```python
from build123d import *

# Parameters (mm, degrees)
SKETCH1_R           = 1.5
BOSS_EXTRUDE1_DEPTH = 2


with BuildPart() as part:
    # Sketch1 → Boss-Extrude1 (new body)
    with BuildSketch(Plane.XY):
        with BuildLine():
            Line((0, 0), (0, 18))
            Line((0, 18), (4, 17.99998836))
            Line((4, 17.99998836), (3.999996862, 13.99998836))
            Line((3.999996862, 13.99998836), (9.631513212, 13.99998836))
            Line((9.631513212, 13.99998836), (9.631513212, 17.99998836))
            Line((9.631513212, 17.99998836), (26.920387768, 13.248592057))
            ThreePointArc((26.920387768, 13.248592057), (31.81744671, 5.842881132), (25.13296029, -0.000352724))
            Line((25.13296029, -0.000352724), (9.631467627, -0.000352724))
            Line((9.631467627, -0.000352724), (9.631467627, 3.999647276))
            Line((9.631467627, 3.999647276), (4, 3.999647276))
            Line((4, 3.999647276), (4, 0))
            Line((4, 0), (0, 0))
        make_face()
        with Locations((25.13296029, 6.744691419)):
            Circle(SKETCH1_R, mode=Mode.SUBTRACT)
        Polygon((14.250450019, 12.02557168), (12.280834513, 11.678275325), (13.149075402, 6.75423656), (15.118690908, 7.101532915), align=None, mode=Mode.SUBTRACT)
        Polygon((7.356795748, 10.810034437), (8.225036637, 5.885995672), (6.255421131, 5.538699316), (5.387180242, 10.462738081), align=None, mode=Mode.SUBTRACT)
    extrude(amount=BOSS_EXTRUDE1_DEPTH)


solid = part.part
```
The listing builds one solid part. Answer for the finished solid, in the listing's coordinates (mm). A direction names the side the tool comes from. Coordinates: 2 decimals unless noted, no trailing zeros. Loops run counter-clockwise (first coordinate to the right, second up) from the corner with the lowest first, then second, coordinate; pieces in that order, holes last. Notation, with made-up numbers: (-38.5, 4.25) - (3.5, 4.25) arc R5 ccw to (3.5, 13.25) - close; hole circle Ø8 at (-37, -1). An arc over 180 degrees is marked (long way). Use a Markdown table: item, result. Add a question column.
1) The part is cut by section B-B, the plane y = 3.25. Give the vertices of the cut face in (x, z).
2) The part is cut by section A-A, the plane x = 25.5. Give the vertices of the cut face in (y, z).
3) The part is cut by section D-D, the plane x = 15.5. Give the vertices of the cut face in (y, z), and give its area (3 significant figures).
4) Find the intervals of material crossed by line 1 (X direction, y = 10.25, z = 0.75); line 2 (X direction, y = 9.25, z = 1.75); line 3 (X direction, y = 8, z = 0.35), in increasing order.
5) The part is cut by section C-C, the plane z = 0.7. Give the vertices of the cut face in (x, y).
6) The mould has two halves that part along Y. Classify faces 1 (the flat face through (7.254, 5.715, 0.986)), 2 (the cylindrical face through (31.834, 5.978, 0.986)), 3 (the flat face through (17, 0, 1)): released by +Y, released by -Y, zero draft, split by the parting line, or undercut.
7) Given pin 1 (1 mm diameter, centred on x = 6, z = 1, fed in from +Y); pin 2 (0.6 mm diameter, centred on y = 1.5, z = 1, fed in from +X); pin 3 (2.5 mm diameter, centred on x = 25.13, y = 6.74, fed in from +Z), each flat-ended and moving along its own axis, determine where each tip first touches the part or whether it passes through.
8) For faces 4 (the flat face through (9.631, 2, 1)), 5 (the flat face through (0, 9, 1)), 6 (the flat face through (9.632, 16, 1)), 7 (the flat face through (7.785, 8.382, 0.986)), determine the directions among +Z, -Z, +X, -X, +Y, -Y from which every point of the face is accessible in a straight line to the end or side of a thin tool.
Here are the results:
| question | item | result |
|---|---|---|
| 1 | outline | (0, 0) - (4, 0) - (4, 2) - (0, 2) - close; (9.63, 0) - (30.9, 0) - (30.9, 2) - (9.63, 2) - close |
| 2 | outline | (0.01, 0) - (5.29, 0) - (5.29, 2) - (0.01, 2) - close; (8.2, 0) - (13.64, 0) - (13.64, 2) - (8.2, 2) - close |
| 3 | outline | (0, 0) - (16.39, 0) - (16.39, 2) - (0, 2) - close |
| 3 | area | 32.8 mm^2 |
| 4 | line 1 | x = 0 to 5.42, 7.46 to 12.53, 14.56 to 30.9 |
| 4 | line 2 | x = 0 to 5.6, 7.63 to 12.71, 14.74 to 31.4 |
| 4 | line 3 | x = 0 to 5.82, 7.85 to 12.93, 14.96 to 24.31, 25.95 to 31.76 |
| 5 | outline | (0, 0) - (4, 0) - (4, 4) - (9.63, 4) - (9.63, 0) - (25.13, 0) arc R6.75 ccw to (26.92, 13.25) - (9.63, 18) - (9.63, 14) - (4, 14) - (4, 18) - (0, 18) - close; hole (5.39, 10.46) - (6.26, 5.54) - (8.23, 5.89) - (7.36, 10.81) - close; hole (12.28, 11.68) - (13.15, 6.75) - (15.12, 7.1) - (14.25, 12.03) - close; hole circle Ø3 at (25.13, 6.74) |
| 6 | face 1 | undercut |
| 6 | face 2 | split by the parting line |
| 6 | face 3 | released by -Y |
| 7 | pin 1 | stops at y = 14 |
| 7 | pin 2 | stops at x = 29.72 |
| 7 | pin 3 | passes through |
| 8 | face 4 | +Z, -Z, -Y |
| 8 | face 5 | +Z, -Z, -X, +Y, -Y |
| 8 | face 6 | +Z, -Z, +Y |
| 8 | face 7 | +Z, -Z |
